```python
from build123d import *

# Parameters (mm, degrees)
BOSS_EXTRU_1_DEPTH = 4.900038


with BuildPart() as part:
    # Esquisse1 → Boss.-Extru.1 (new body)
    with BuildSketch(Plane.XZ):
        with BuildLine():
            Line((-0.815337621, 41.120678267), (-0.815337621, 34.249109833))
            ThreePointArc((-0.815337621, 34.249109833), (-0.229551316, 32.834896593), (1.184661924, 32.249110289))
            Line((1.184661924, 32.249110289), (7.484661488, 32.249110289))
            ThreePointArc((7.484661488, 32.249110289), (8.898874021, 31.663324278), (9.484660032, 30.249111745))
            Line((9.484660032, 30.249111745), (9.484660032, 21.610522714))
            ThreePointArc((9.484660032, 21.610522714), (9.236435528, 20.794530717), (8.575860046, 20.254995384))
            Line((8.575860046, 20.254995384), (6.723618468, 19.851925476))
            Line((6.723618468, 19.851925476), (4.953621871, 19.173415631))
            Line((4.953621871, 19.173415631), (3.306576246, 18.235075845))
            Line((3.306576246, 18.235075845), (2.706450383, 17.599525989))
            Line((2.706450383, 17.599525989), (2.434698445, 16.768726179))
            Line((2.434698445, 16.768726179), (2.54322942, 15.901386376))
            Line((2.54322942, 15.901386376), (3.011310314, 15.163166545))
            Line((3.011310314, 15.163166545), (4.654204939, 13.520266919))
            Line((4.654204939, 13.520266919), (4.868308891, 13.393666948))
            Line((4.868308891, 13.393666948), (5.116923834, 13.38588695))
            Line((5.116923834, 13.38588695), (5.338521783, 13.498866924))
            ThreePointArc((5.338521783, 13.498866924), (15.463306351, 11.777438967), (14.377512906, 1.564915804))
            ThreePointArc((14.377512906, 1.564915804), (14.224756538, 1.21764125), (14.398922901, 0.88059496))
            Line((14.398922901, 0.88059496), (16.041812526, -0.762298665))
            ThreePointArc((16.041812526, -0.762298665), (17.647380358, -1.33891093), (19.113721826, -0.467032233))
            Line((19.113721826, -0.467032233), (20.286561559, 1.706666772))
            Line((20.286561559, 1.706666772), (21.009101394, 4.068549234))
            Line((21.009101394, 4.068549234), (21.253121339, 6.526390674))
            Line((21.253121339, 6.526390674), (21.253121339, 15.699105144))
            ThreePointArc((21.253121339, 15.699105144), (21.106674763, 16.052658454), (20.753121453, 16.19910503))
            Line((20.753121453, 16.19910503), (16.687787672, 16.19910503))
            ThreePointArc((16.687787672, 16.19910503), (16.261005783, 16.022326184), (16.43778463, 16.449108073))
            Line((16.43778463, 16.449108073), (16.43778463, 20.849107628))
            ThreePointArc((16.43778463, 20.849107628), (16.261009771, 21.275879889), (16.687782032, 21.09910503))
            Line((16.687782032, 21.09910503), (27.937782009, 21.09910503))
            ThreePointArc((27.937782009, 21.09910503), (28.291335319, 21.245551606), (28.437781895, 21.599104916))
            Line((28.437781895, 21.599104916), (28.437781895, 37.999105144))
            ThreePointArc((28.437781895, 37.999105144), (28.291335319, 38.352658454), (27.937782009, 38.49910503))
            Line((27.937782009, 38.49910503), (16.687785131, 38.49910503))
            ThreePointArc((16.687785131, 38.49910503), (16.26100758, 38.322327981), (16.43778463, 38.749105532))
            Line((16.43778463, 38.749105532), (16.43778463, 43.14910503))
            ThreePointArc((16.43778463, 43.14910503), (16.261007934, 43.575881726), (16.68778463, 43.39910503))
            Line((16.68778463, 43.39910503), (20.753121453, 43.39910503))
            ThreePointArc((20.753121453, 43.39910503), (21.106674763, 43.545551606), (21.253121339, 43.899104916))
            Line((21.253121339, 43.899104916), (21.253121339, 51.526382419))
            Line((21.253121339, 51.526382419), (21.824434721, 54.609591947))
            Line((21.824434721, 54.609591947), (21.833435025, 57.694186853))
            Line((21.833435025, 57.694186853), (19.84525724, 59.242523707))
            Line((19.84525724, 59.242523707), (19.209707385, 59.84265357))
            Line((19.209707385, 59.84265357), (18.378917574, 60.114403508))
            Line((18.378917574, 60.114403508), (17.511567772, 60.005873533))
            Line((17.511567772, 60.005873533), (16.77334794, 59.537793639))
            Line((16.77334794, 59.537793639), (15.130452537, 57.894888236))
            ThreePointArc((15.130452537, 57.894888236), (14.984254305, 57.556974361), (15.109048319, 57.21058417))
            ThreePointArc((15.109048319, 57.21058417), (14.787965349, 46.945806953), (4.52318847, 46.624713214))
            ThreePointArc((4.52318847, 46.624713214), (4.176789338, 46.749509832), (3.838867319, 46.603307018))
            Line((3.838867319, 46.603307018), (-0.229554407, 42.534884292))
            ThreePointArc((-0.229554407, 42.534884292), (-0.663097525, 41.886041033), (-0.815337621, 41.120678267))
        make_face()
        with BuildLine():
            Line((9.484660032, 37.259480615), (9.484660032, 35.749109175))
            ThreePointArc((9.484660032, 35.749109175), (9.338213749, 35.395556572), (8.984661146, 35.249110289))
            Line((8.984661146, 35.249110289), (3.684660032, 35.249110289))
            ThreePointArc((3.684660032, 35.249110289), (3.331106642, 35.395556899), (3.184660032, 35.749110289))
            Line((3.184660032, 35.749110289), (3.184660032, 38.615420306))
            ThreePointArc((3.184660032, 38.615420306), (3.421541448, 39.040593437), (3.907737867, 39.062910204))
            Line((3.907737867, 39.062910204), (6.386454303, 38.139900415))
            Line((6.386454303, 38.139900415), (9.003891164, 37.759110289))
            ThreePointArc((9.003891164, 37.759110289), (9.329866443, 37.591655279), (9.484660032, 37.259480615))
        make_face(mode=Mode.SUBTRACT)
    extrude(amount=-BOSS_EXTRU_1_DEPTH)


solid = part.part
```
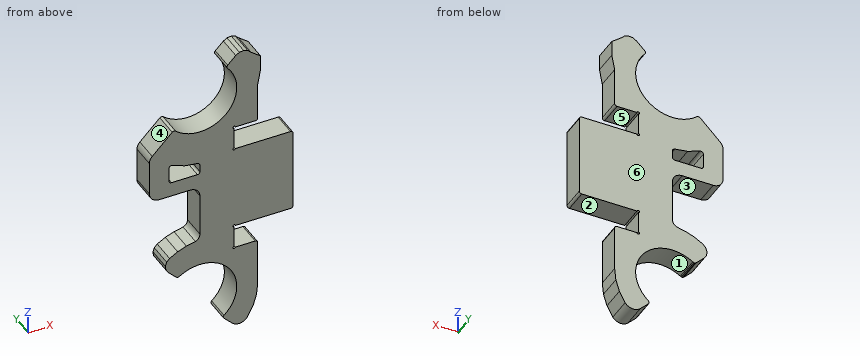
The listing builds one solid part. Answer for the finished solid, in the listing's coordinates (mm). Face numbers are marked on the shaded views. A direction names the side the tool comes from. Round coordinates to 2 decimals unless told otherwise and drop trailing zeros. Loops run counter-clockwise (first coordinate to the right, second up) from the corner with the lowest first, then second, coordinate; pieces in that order, holes last. Notation, with made-up numbers: (36.25, 68) - (56.25, 68) arc R14 ccw to (56.25, 83) - close; hole circle Ø2 at (5, 53.5). An arc over 180 degrees is marked (long way). Return JSON: item names as keys, results as strings. Group by question number.
1. Consider probe 1 along Z at (x, y) = (17.5, 2.15); probe 2 along Z at (x, y) = (5.5, 0.65); probe 3 along X at (y, z) = (3.45, 24). Determine where each line is inside the solid, lowest interval first.
2. Each of these flat-tipped pins is pushed along its axis until it touches: P1, Ø1.3, axis at y = 3, z = 19, coming from the +X side; P2, Ø1.5, axis at y = 1.5, z = 47.5, coming from the +X side; P3, Ø2.5, axis at x = 7, y = 2.5, coming from the +Z side. Where does it stop, or does it pass through?
3. The part is cut by section A-A on z = 36.5. Determine the outline of the cut face in (x, y), then the cut area to 3 significant figures.
4. The mould has two halves that part along Z. Classify the marked faces 4, 5 and 6: pulls with the +Z half, pulls with the -Z half, needs draft (parallel to the pull), parting line crosses it, or undercut.
5. The part is cut by section C-C on x = 25.25. Determine the outline of the cut face in (y, z), then the cut area to 3 significant figures.
6. The part is cut by section B-B on z = 25. Determine the outline of the cut face in (x, y), then the cut area to 3 significant figures.
7. Which of the six approach directions +Z, -Z, +X, -X, +Y, -Y give full straight-line access (tool end or side, diameter ignored) to the marked faces 1, 2 and 3?
Resolved:
{
 "1": {"probe 1": "z = -1.35 to 16.2, 21.1 to 38.5, 43.4 to 60", "probe 2": "z = 13.6 to 19.38, 32.25 to 35.25, 38.47 to 45.9", "probe 3": "x = 9.48 to 28.44"},
 "2": {"P1": "stops at x = 16.44", "P2": "stops at x = 21.25", "P3": "stops at z = 45.75"},
 "3": {"outline": "(-0.82, 0) - (3.18, 0) - (3.18, 4.9) - (-0.82, 4.9) - close; (9.48, 0) - (28.44, 0) - (28.44, 4.9) - (9.48, 4.9) - close", "area": "112 mm²"},
 "4": {"face 4": "pulls with the +Z half", "face 5": "undercut", "face 6": "needs draft"},
 "5": {"outline": "(0, 21.1) - (4.9, 21.1) - (4.9, 38.5) - (0, 38.5) - close", "area": "85.3 mm²"},
 "6": {"outline": "(9.48, 0) - (28.44, 0) - (28.44, 4.9) - (9.48, 4.9) - close", "area": "92.9 mm²"},
 "7": {"face 1": "+Y, -Y", "face 2": "+X, +Y, -Y", "face 3": "-X, +Y, -Y"}
}
